Design review of the part built by this model. Coordinates are the model's own, in mm. Give positions to 0.01 mm unless a question says otherwise; leave off trailing zeros. Write each question's results on one line, items separated by ' | '.
```python
from build123d import *

# Parameters (mm, degrees)
F1_DEPTH = 620


with BuildPart() as f1:
    # F0 (on Front) → F1 (new body)
    with BuildSketch(Plane.XZ):
        Polygon((5, -20), (20, -20), (20, -5), (15, -5), (15, -10), (10, -5), (10, 5), (15, 10), (15, 5), (20, 5), (20, 20), (20, 35), (15, 35), (15, 30), (10, 35), (10, 45), (15, 50), (15, 45), (20, 45), (20, 60), (5, 60), (5, 55), (10, 55), (5, 50), (-5, 50), (-10, 55), (-5, 55), (-5, 60), (-20, 60), (-20, 45), (-15, 45), (-15, 50), (-10, 45), (-10, 35), (-15, 30), (-15, 35), (-20, 35), (-20, 20), (-20, 5), (-15, 5), (-15, 10), (-10, 5), (-10, -5), (-15, -10), (-15, -5), (-20, -5), (-20, -20), (-5, -20), (-5, -15), (-10, -15), (-5, -10), (5, -10), (10, -15), (5, -15), align=None)
        Polygon((-5, 0), (-5, 5), (0, 5), (5, 5), (5, 0), (5, -5), (0, -5), (-5, -5), align=None, mode=Mode.SUBTRACT)
        Polygon((-5, 15), (-5, 20), (-5, 25), (-10, 25), (-5, 30), (5, 30), (10, 25), (5, 25), (5, 20), (5, 15), (10, 15), (5, 10), (-5, 10), (-10, 15), align=None, mode=Mode.SUBTRACT)
        Polygon((-5, 40), (-5, 45), (0, 45), (5, 45), (5, 40), (5, 35), (0, 35), (-5, 35), align=None, mode=Mode.SUBTRACT)
    extrude(amount=F1_DEPTH)


solid = f1.part
```
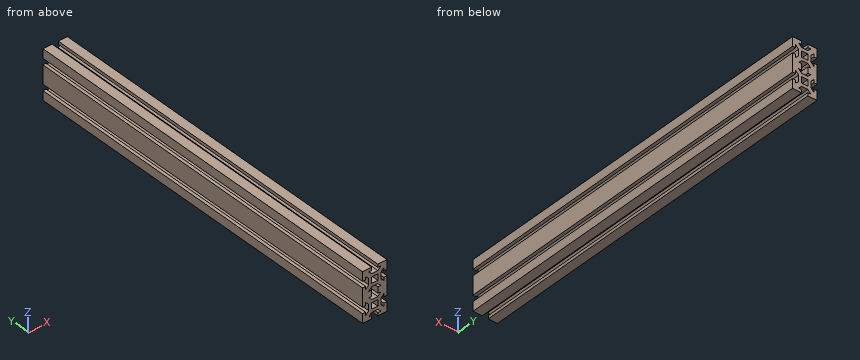
Item 1: Clearance check with flat-ended pins moving along their axes: P1, Ø4, axis at x = -8.5, z = 10, coming from the +Y side; P2, Ø5, axis at y = -162.5, z = 40, coming from the -X side; P3, Ø1.5, axis at y = -437.5, z = 44, coming from the +X side; P4, Ø5, axis at x = 2, y = -268, coming from the +Z side. State where each tip first meets the part, or that it passes through.
Output values:
P1: stops at y = 0 | P2: stops at x = -10 | P3: stops at x = 10 | P4: stops at z = 50
Item 2: We need section A-A on y = -300. Give the number of separate pieces and of enclosed holes in the cut face, then the cut area to 3 significant figures.
Output values:
separate pieces: 1 | enclosed holes: 3 | area: 2,000 mm²
Item 3: Wall thickness on probe 1 along Z at (x, y) = (4, -29.5); probe 2 along Z at (x, y) = (-16.5, -450.5); probe 3 along X at (y, z) = (-558, 8.5): over which ranges is each line inside the solid? List them lowest first.
Output values:
probe 1: z = -10 to -5, 5 to 10, 30 to 35, 45 to 50 | probe 2: z = -20 to -5, 5 to 35, 45 to 60 | probe 3: x = -20 to -15, -13.5 to 13.5, 15 to 20
